The model under review builds one solid part; all positions refer to its coordinate system, in mm. Give positions to 0.01 mm unless a question says otherwise; leave off trailing zeros. Order: outer loops, then holes, each group sorted by start corner. A loop starts at its lowest first (then second) coordinate and runs counter-clockwise, first axis right, second up. Notation, with made-up numbers: (-26.75, -11) - (-17.75, -11) arc R32 cw to (-17.75, 26) - close; hole circle Ø2 at (-24, -31.5). An arc over 180 degrees is marked (long way). Answer as CSV lines item,"result". Start each with the question number.
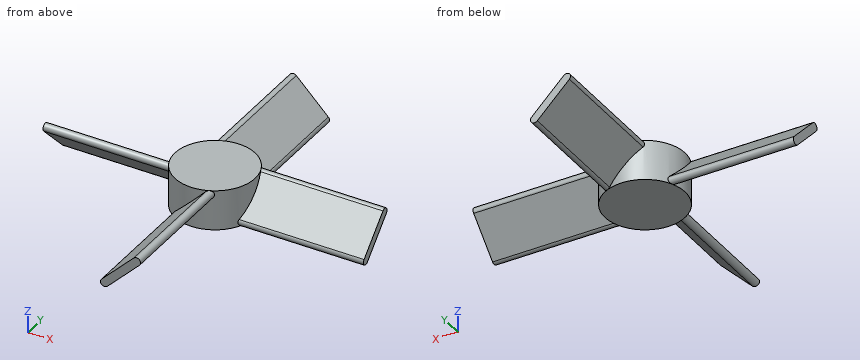
from build123d import *

# Parameters (mm, degrees)
F0_R     = 12.7
F1_DEPTH = 6.35
F3_DEPTH = 50.8
F4_COUNT = 4


with BuildPart() as f1:
    # F0 (on Top) → F1 (new body, symmetric)
    with BuildSketch(Plane.XY):
        Circle(F0_R)
    extrude(amount=F1_DEPTH, both=True)

    # F2 (on Right) → F3 (join)
    with BuildSketch(Plane.YZ):
        with BuildLine():
            Line((-4.1819743879, -5.9780256121), (5.9780256121, 4.1819743879))
            ThreePointArc((5.9780256121, 4.1819743879), (5.9780256121, 5.9780256121), (4.1819743879, 5.9780256121))
            Line((4.1819743879, 5.9780256121), (-5.9780256121, -4.1819743879))
            ThreePointArc((-5.9780256121, -4.1819743879), (-5.9780256121, -5.9780256121), (-4.1819743879, -5.9780256121))
        make_face()
    extrude(amount=F3_DEPTH)

    # F4: F1 ×4 about axis
    f4_axis = Axis((0, 0, 0), (0, 0, 1))


with BuildPart() as f1_1:
    add(f1.part)
    for i in range(1, F4_COUNT):
        add(f1.part.rotate(f4_axis, i * 360 / F4_COUNT))


solid = f1_1.part
Item 1: For line 1 along Z through (x, y) = (-34, -6); line 2 along Y through (x, z) = (11, -3.5); line 3 along Y through (x, z) = (-13.5, 3.25), list the stretches that pass through material, from the lowest coordinate up.
Item 2: Take a section at A-A on y = -34.5. Write out the cut boundary in (x, z), and give its area (3 significant figures).
Item 3: Clearance check with flat-ended pins moving along their axes: pin 1 (3 mm diameter, centred on y = 27, z = 4.5, fed in from -X); pin 2 (4 mm diameter, centred on y = 29, z = 0, fed in from +X); pin 3 (2 mm diameter, centred on x = -16.5, z = -0.5, fed in from +Y). State where each tip first meets the part, or that it passes through.
Item 4: Take a section at B-B on z = -0.25. Write out the cut boundary in (x, y).
Data:
1,line 1,"z = 4.2 to 5.96"
1,line 2,"y = -6.35 to 6.35"
1,line 3,"y = -5.05 to -1.45"
2,outline,"(-5.98, -4.18) arc R1.27 ccw to (-4.18, -5.98) - (5.98, 4.18) arc R1.27 ccw to (4.18, 5.98) - close"
2,area,"41.6 mm^2"
3,pin 1,"stops at x = -6.35"
3,pin 2,"stops at x = 3.8"
3,pin 3,"stops at y = 3.3"
4,outline,"(-50.8, -1.55) - (-12.61, -1.55) arc R12.7 ccw to (-2.05, -12.53) - (-2.05, -50.8) - (1.55, -50.8) - (1.55, -12.61) arc R12.7 ccw to (12.53, -2.05) - (50.8, -2.05) - (50.8, 1.55) - (12.61, 1.55) arc R12.7 ccw to (2.05, 12.53) - (2.05, 50.8) - (-1.55, 50.8) - (-1.55, 12.61) arc R12.7 ccw to (-12.53, 2.05) - (-50.8, 2.05) - close"
